For this review, use the dimensioned drawing (mm, ordinates from the lowest corner) and the shaded views. Coordinates: 2 decimals unless noted, no trailing zeros. Order: outer loops, then holes, each group sorted by start corner. A loop starts at its lowest first (then second) coordinate and runs counter-clockwise, first axis right, second up. Notation, with made-up numbers: (57.5, -12) -> (91.5, -12) arc R21 cw to (91.5, 13) -> close; hole circle Ø8 at (79.25, 28.5). An arc over 180 degrees is marked (long way). Use one line per item in the form item = value. Start each with the question number.
(1) Mouldability with a two-part tool opening along Z and no side actions: class the marked faces 1, 2, 3 and 4 as +Z half, -Z half, draft (parallel to the pull), parting line (faces both ways), or undercut.
(2) Take a section at D-D (z = 3). State the section outline as (x, y) points.
(3) Insertion check: pin 1 Ø3.5 at (x, z) = (4.5, 7.5) entering from -Y; pin 2 Ø5 at (x, z) = (37.5, 7.5) entering from -Y; pin 3 Ø1.2 at (y, z) = (5, 1.5) entering from +X; pin 4 Ø1.2 at (y, z) = (3, 1) entering from -X. Each pin has a flat end and moves straight along its axis. Give the tip position at first contact, or say it passes through.
(4) Take a section at A-A (y = 5.5). State the section outline as (x, z) points.
(5) Wall thickness on line 1 along X through (y, z) = (2.75, 6.5); line 2 along X through (y, z) = (1, 6.25); line 3 along X through (y, z) = (7, 10.75): over which ranges is each line inside the solid? List them lowest first.
(6) Take a section at C-C (x = 4.5). State the section outline as (y, z) points, then the cut area to 3 significant figures.
(7) Take a section at B-B (z = 7.5). State how many separate pieces and enclosed holes the cut face has, then the cut area to 3 significant figures.
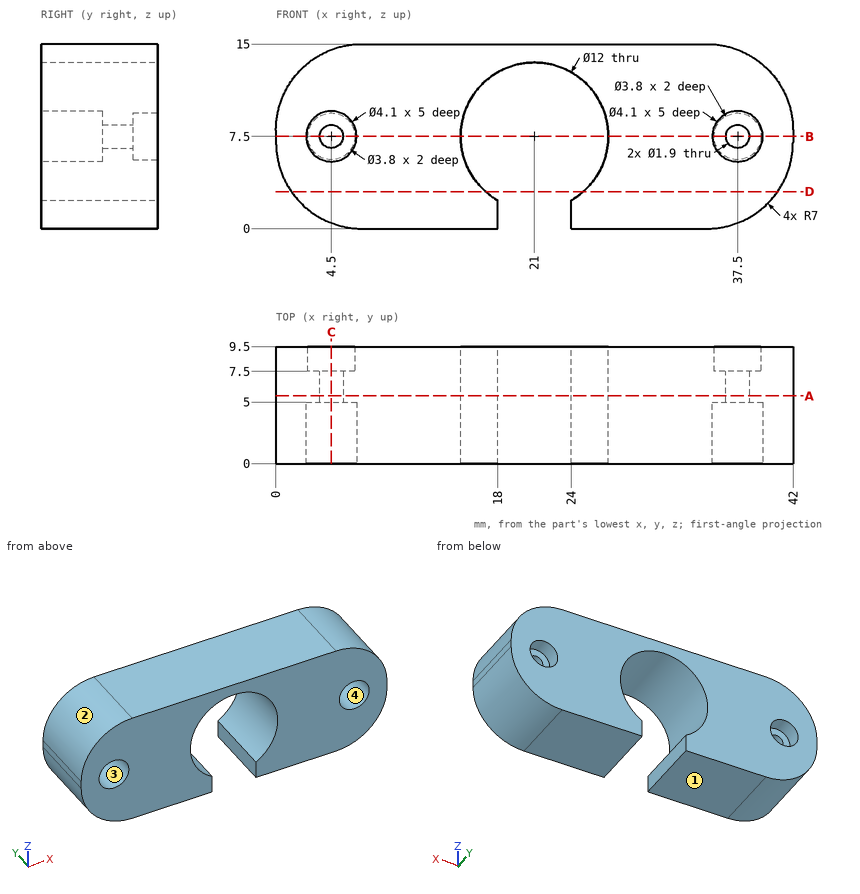
Findings:
q1.face_1 = -Z half
q1.face_2 = +Z half
q1.face_3 = undercut
q1.face_4 = undercut
q2.outline = (1.26, 0) -> (17.03, 0) -> (17.03, 9.5) -> (1.26, 9.5) -> close; (24.97, 0) -> (40.74, 0) -> (40.74, 9.5) -> (24.97, 9.5) -> close
q3.pin_1 = 5
q3.pin_2 = 0
q3.pin_3 = 40
q3.pin_4 = 2.55
q4.outline = (0, 7) arc R7 ccw to (7, 0) -> (18, 0) -> (18, 2.3) arc R6 cw (long way) to (24, 2.3) -> (24, 0) -> (35, 0) arc R7 ccw to (42, 7) -> (42, 8) arc R7 ccw to (35, 15) -> (7, 15) arc R7 ccw to (0, 8) -> close; hole circle Ø1.9 at (4.5, 7.5); hole circle Ø1.9 at (37.5, 7.5)
q5.line_1 = 0.02 to 2.71, 6.29 to 15.08, 26.92 to 35.71, 39.29 to 41.98
q5.line_2 = 0.04 to 2.88, 6.12 to 15.13, 26.87 to 35.88, 39.12 to 41.96
q5.line_3 = 0.56 to 15.96, 26.04 to 41.44
q6.outline = (0, 0.46) -> (9.5, 0.46) -> (9.5, 5.6) -> (7.5, 5.6) -> (7.5, 6.55) -> (5, 6.55) -> (5, 5.45) -> (0, 5.45) -> close; (0, 9.55) -> (5, 9.55) -> (5, 8.45) -> (7.5, 8.45) -> (7.5, 9.4) -> (9.5, 9.4) -> (9.5, 14.54) -> (0, 14.54) -> close
q6.area = 101 mm²
q7.separate_pieces = 4
q7.enclosed_holes = 0
q7.area = 219 mm²
